Can you work these out from the model? Positions are in its coordinate system, mm. Coordinates: 2 decimals unless noted, no trailing zeros. Loops run counter-clockwise (first coordinate to the right, second up) from the corner with the lowest first, then second, coordinate; pieces in that order, holes last. Notation, with made-up numbers: M 59,68 L 115,68 A33 cw 115,96 Z; hole C -20,34.5 d1. An arc over 180 degrees is marked long. Answer as a JSON object with one key per item and string values. Group by question number.
Item 1: Suppose I cut it at B-B (z = 3.65). Count the separate pieces of the cut face and the enclosed holes in it, then the cut area to 3 significant figures.
Item 2: Suppose I cut it at C-C (x = -125.5). Write out the boundary of the cut face in (y, z).
Item 3: Suppose I cut it at A-A (x = -90). Write out the boundary of the cut face in (y, z).
Item 4: I'm going to push flat-ended pins straight in: pin 1 Ø2 at (y, z) = (-131, 3) entering from +X; pin 2 Ø3 at (y, z) = (-182, 3) entering from -X; pin 3 Ø1.5 at (y, z) = (-234, 2) entering from -X. Where does each tip first touch, or does it pass through?
Item 5: If I drill on line 1 (X direction, y = -170, z = 3.1); line 2 (Y direction, x = -90, z = 3.9); line 3 (Y direction, x = -65, z = 2.4), over which ranges is the centre line in solid material (lowest first)?
```python
from build123d import *

# Parameters (mm, degrees)
MODEL_R                  = 1.5
MODEL_R_2                = 2.5
RESSALTO_EXTRUS_O1_DEPTH = 6


with BuildPart() as part:
    # Model → Ressalto-extrusão1 (new body)
    with BuildSketch(Plane.XY):
        Polygon((-5, -175), (0, -175), (0, -165), (-5, -165), (-5, -155), (0, -155), (0, -45), (-5, -45), (-5, -35), (0, -35), (0, -25), (-5, -25), (-5, -15), (0, -15), (0, 0), (-25, 0), (-25, -5), (-35, -5), (-35, 0), (-45, 0), (-45, -5), (-55, -5), (-55, 0), (-145, 0), (-145, -5), (-155, -5), (-155, 0), (-165, 0), (-165, -5), (-175, -5), (-175, 0), (-200, 0), (-200, -15), (-195, -15), (-195, -25), (-200, -25), (-200, -35), (-195, -35), (-195, -45), (-200, -45), (-200, -155), (-195, -155), (-195, -165), (-200, -165), (-200, -175), (-195, -175), (-195, -185), (-200, -185), (-200, -200.74174754), (-190.853525683, -209.17356867), (-188.481322389, -206.600305295), (-181.128851073, -213.378296557), (-183.501054367, -215.951559933), (-176.501501675, -222.404207614), (-174.096972592, -219.795878624), (-166.741593597, -226.576550376), (-169.14612268, -229.184879366), (-159.999648363, -237.616700496), (-150, -237.53283976), (-150, -232.5), (-140, -232.5), (-140, -237.5), (-130, -237.5), (-130, -232.5), (-120, -232.5), (-120, -237.5), (-80, -237.5), (-80, -232.5), (-70, -232.5), (-70, -237.5), (-60, -237.5), (-60, -232.5), (-50, -232.5), (-50, -237.5), (-40.000351637, -237.583860737), (-30.85387732, -229.152039608), (-33.759891511, -225.999721294), (-26.407420195, -219.221730032), (-23.852117489, -221.993611718), (-16.496373021, -215.21260305), (-19.051675727, -212.440721364), (-11.69920441, -205.662730102), (-9.146474317, -208.43182113), (0, -200), (0, -185), (-5, -185), align=None)
        with Locations((-2.5, -170)):
            Circle(MODEL_R, mode=Mode.SUBTRACT)
        with Locations((-2.5, -30)):
            Circle(MODEL_R, mode=Mode.SUBTRACT)
        with Locations((-40, -2.5)):
            Circle(MODEL_R, mode=Mode.SUBTRACT)
        with Locations((-160, -2.5)):
            Circle(MODEL_R, mode=Mode.SUBTRACT)
        with Locations((-197.5, -30)):
            Circle(MODEL_R, mode=Mode.SUBTRACT)
        with Locations((-197.5, -170)):
            Circle(MODEL_R, mode=Mode.SUBTRACT)
        with Locations((-65, -235)):
            Circle(MODEL_R, mode=Mode.SUBTRACT)
        with Locations((-135, -235)):
            Circle(MODEL_R, mode=Mode.SUBTRACT)
        with Locations((-90, -52.5)):
            Circle(MODEL_R_2, mode=Mode.SUBTRACT)
        with Locations((-110, -12.5)):
            Circle(MODEL_R_2, mode=Mode.SUBTRACT)
        with Locations((-90, -12.5)):
            Circle(MODEL_R_2, mode=Mode.SUBTRACT)
        with Locations((-110, -52.5)):
            Circle(MODEL_R_2, mode=Mode.SUBTRACT)
        with Locations((-178.608483127, -218.05063468)):
            Circle(MODEL_R, mode=Mode.SUBTRACT)
        with Locations((-21.21191866, -217.474200234)):
            Circle(MODEL_R, mode=Mode.SUBTRACT)
        with BuildLine():
            Line((-56.5, -55), (-56.5, -45))
            ThreePointArc((-56.5, -45), (-55, -43.5), (-53.5, -45))
            Line((-53.5, -45), (-53.5, -55))
            ThreePointArc((-53.5, -55), (-55, -56.5), (-56.5, -55))
        make_face(mode=Mode.SUBTRACT)
        with BuildLine():
            Line((-53.5, -75), (-53.5, -85))
            ThreePointArc((-53.5, -85), (-55, -86.5), (-56.5, -85))
            Line((-56.5, -85), (-56.5, -75))
            ThreePointArc((-56.5, -75), (-55, -73.5), (-53.5, -75))
        make_face(mode=Mode.SUBTRACT)
        with BuildLine():
            Line((-146.5, -85), (-146.5, -75))
            ThreePointArc((-146.5, -75), (-145, -73.5), (-143.5, -75))
            Line((-143.5, -75), (-143.5, -85))
            ThreePointArc((-143.5, -85), (-145, -86.5), (-146.5, -85))
        make_face(mode=Mode.SUBTRACT)
        with BuildLine():
            Line((-146.5, -55), (-146.5, -45))
            ThreePointArc((-146.5, -45), (-145, -43.5), (-143.5, -45))
            Line((-143.5, -45), (-143.5, -55))
            ThreePointArc((-143.5, -55), (-145, -56.5), (-146.5, -55))
        make_face(mode=Mode.SUBTRACT)
    extrude(amount=RESSALTO_EXTRUS_O1_DEPTH)


solid = part.part
```
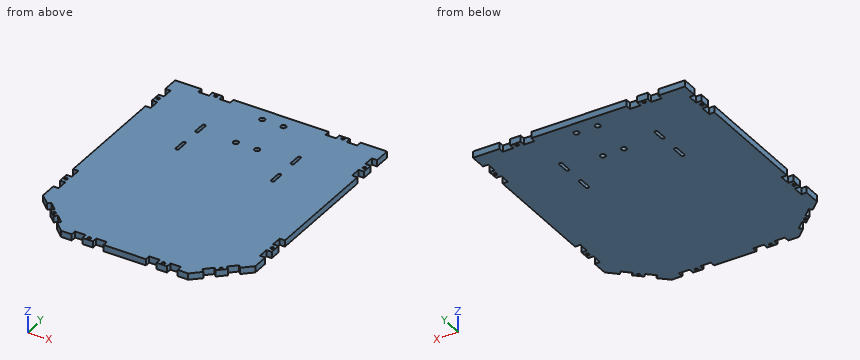
From the geometry:
{
 "1": {"separate pieces": "1", "enclosed holes": "18", "area": "44,800 mm2"},
 "2": {"outline": "M -232.5,0 L 0,0 L 0,6 L -232.5,6 Z"},
 "3": {"outline": "M -237.5,0 L -55,0 L -55,6 L -237.5,6 Z; M -50,0 L -15,0 L -15,6 L -50,6 Z; M -10,0 L 0,0 L 0,6 L -10,6 Z"},
 "4": {"pin 1": "x = 0", "pin 2": "x = -195", "pin 3": "x = -164.74"},
 "5": {"line 1": "-200 to -199, -196 to -4, -1 to 0", "line 2": "-237.5 to -55, -50 to -15, -10 to 0", "line 3": "-237.5 to -236.5, -233.5 to 0"}
}
